Solid Edge part; units mm, degrees
sketch "Sketch1" plane through (0, 0, 0) normal (0, 0, 1) x (1, 0, 0)
  circle A0 centre (0, 0) radius 7.5
extrude "ExtrudedProtrusion_1" add sketch "Sketch1" along normal blind 250 and the other way blind 85
sketch "Sketch2" plane through (0, 0, 0) normal (0, 0, 1) x (1, 0, 0)
  line L0 (-1.5, 6.5) -> (1.5, 6.5)
  line L1 (1.5, 6.5) -> (1.5, 8.5)
  line L2 (1.5, 8.5) -> (-1.5, 8.5)
  line L3 (-1.5, 8.5) -> (-1.5, 6.5)
  dimension "D1" = 1.5
extrude "ExtrudedProtrusion_2" add sketch "Sketch2" along normal blind 30
sketch "Sketch3" plane through (0, 0, 250) normal (0, 0, 1) x (0, 1, 0)
  line L0 (1.5023, 6.5) -> (-1.5023, 6.5)
  line L1 (-1.5023, 6.5) -> (-1.5023, 8.5)
  line L2 (-1.5023, 8.5) -> (1.5023, 8.5)
  line L3 (1.5023, 8.5) -> (1.5023, 6.5)
  dimension "D1" = 1.5023
  dimension "D2" = 1.5023
extrude "ExtrudedProtrusion_3" add sketch "Sketch3" against normal blind 50
properties material "Aluminum, 1060"
Could you check a few things on this model? Use its own coordinates, in mm. Give positions to 0.01 mm unless a question says otherwise; leave off trailing zeros. Write each loop counter-clockwise with the first axis right and the second up, starting at its lowest first coordinate (ties: lowest second). Pieces come first, ordered by that corner, then holes. Notation, with made-up numbers: (-28.5, 54.5) -> (4.5, 54.5) arc R26 cw to (4.5, 79.5) -> close; hole circle Ø7 at (8.5, 63). An arc over 180 degrees is marked (long way). Write each question's results on one line, items separated by ' | '.
1. Will these pins go through, and if not, where does the flat tip stop? pin 1 Ø1.5 at (x, z) = (1, 129.5) entering from +Y; pin 2 Ø0.9 at (y, z) = (8, 17.5) entering from -X; pin 3 Ø6 at (x, z) = (-6.5, 29) entering from +Y.
Check sheet entries:
pin 1: stops at y = 7.5 | pin 2: stops at x = -1.5 | pin 3: stops at y = 6.63
2. I want a section at C-C, the plane z = -24. Write out the boundary of the cut face in (x, y), then the cut area to 3 significant figures.
Check sheet entries:
outline: circle Ø15 at (0, 0) | area: 177 mm²
3. I need wall thicknesses on L1, parallel to Y at x = 0, z = 176; L2, parallel to Y at x = -0.5, z = 24.5; L3, parallel to X at y = -2.25, z = 110.5. Which ranges of each line are inside material? Lowest first, please.
Check sheet entries:
L1: y = -7.5 to 7.5 | L2: y = -7.48 to 8.5 | L3: x = -7.15 to 7.15
4. I want a section at A-A, the plane z = 230. Write out the boundary of the cut face in (x, y).
Check sheet entries:
outline: (-8.5, -1.5) -> (-7.35, -1.5) arc R7.5 ccw (long way) to (-7.35, 1.5) -> (-8.5, 1.5) -> close
5. I want a section at B-B, the plane y = 4.5. Write out the boundary of the cut face in (x, z), then the cut area to 3 significant figures.
Check sheet entries:
outline: (-6, -85) -> (6, -85) -> (6, 250) -> (-6, 250) -> close | area: 4,020 mm²
